from build123d import *

# Parameters (mm, degrees)
SKETCH1_W           = 102.2
SKETCH1_H           = 67.6
SKETCH1_R           = 1.6
BOSS_EXTRUDE1_DEPTH = 6
SKETCH2_W           = 138.2
SKETCH2_H           = 67.6
SKETCH2_R           = 2.5
BOSS_EXTRUDE2_DEPTH = 3.2
FILLET1_R           = 6
FILLET2_R           = 5
FILLET3_R           = 5


with BuildPart() as part:
    # Sketch1 → Boss-Extrude1 (new body)
    with BuildSketch(Plane.XY):
        with Locations((51.1, 33.8)):
            Rectangle(SKETCH1_W, SKETCH1_H)
        with BuildLine():
            Line((94.706674091, 2.5), (7.493325909, 2.5))
            ThreePointArc((7.493325909, 2.5), (7.045584412, 7.045584412), (2.5, 7.493325909))
            Line((2.5, 7.493325909), (2.5, 65.1))
            Line((2.5, 65.1), (99.7, 65.1))
            Line((99.7, 65.1), (99.7, 57.093325909))
            ThreePointArc((99.7, 57.093325909), (94.1, 54.1), (99.7, 51.106674091))
            Line((99.7, 51.106674091), (99.7, 7.493325909))
            ThreePointArc((99.7, 7.493325909), (95.154415588, 7.045584412), (94.706674091, 2.5))
        make_face(mode=Mode.SUBTRACT)
        with Locations((4.5, 4.5)):
            Circle(SKETCH1_R, mode=Mode.SUBTRACT)
        with Locations((97.7, 4.5)):
            Circle(SKETCH1_R, mode=Mode.SUBTRACT)
        with Locations((97.7, 54.1)):
            Circle(SKETCH1_R, mode=Mode.SUBTRACT)
    extrude(amount=BOSS_EXTRUDE1_DEPTH)

    # Sketch2 → Boss-Extrude2 (add)
    with BuildSketch(Plane(origin=(0, 0, 0), x_dir=(-1, 0, 0), z_dir=(0, 0, -1))):
        with Locations((-51.1, 33.8)):
            Rectangle(SKETCH2_W, SKETCH2_H)
        with Locations((-112.2, 59.6)):
            Circle(SKETCH2_R, mode=Mode.SUBTRACT)
        with Locations((-112.2, 8)):
            Circle(SKETCH2_R, mode=Mode.SUBTRACT)
        with Locations((10, 8)):
            Circle(SKETCH2_R, mode=Mode.SUBTRACT)
        with Locations((10, 59.6)):
            Circle(SKETCH2_R, mode=Mode.SUBTRACT)
    extrude(amount=BOSS_EXTRUDE2_DEPTH)

    # Fillet1
    fillet1_edges = [part.edges().sort_by_distance(p)[0] for p in [
        (120.2, 67.6, -1.6),
        (120.2, 0, -1.6),
        (-18, 0, -1.6),
        (-18, 67.6, -1.6),
    ]]
    fillet(fillet1_edges, radius=FILLET1_R)

    # Fillet2
    fillet2_edges = [part.edges().sort_by_distance(p)[0] for p in [
        (99.7, 51.106674091, 3),
        (99.7, 57.093325909, 3),
    ]]
    fillet(fillet2_edges, radius=FILLET2_R)

    # Fillet3
    fillet3_edges = [part.edges().sort_by_distance(p)[0] for p in [
        (7.493325909, 2.5, 3),
        (94.706674091, 2.5, 3),
        (99.7, 7.493325909, 3),
        (2.5, 7.493325909, 3),
    ]]
    fillet(fillet3_edges, radius=FILLET3_R)


solid = part.part
CAD build for the part. Positions are in the model's coordinates, mm. A direction names the side the tool comes from. Round coordinates to 2 decimals unless told otherwise and drop trailing zeros. Order: outer loops, then holes, each group sorted by start corner. A loop starts at its lowest first (then second) coordinate and runs counter-clockwise, first axis right, second up. Notation, with made-up numbers: M 55.5,34 L 96.5,34 A23 ccw 96.5,70 Z; hole C 31,-3 d11. An arc over 180 degrees is marked long. Use one line per item in the form item = value.
Q1. Saw through at A-A on x = -10. Give the cut face in (y, z).
Recorded:
outline = M 0,-3.2 L 5.5,-3.2 L 5.5,0 L 0,0 Z; M 10.5,-3.2 L 57.1,-3.2 L 57.1,0 L 10.5,0 Z; M 62.1,-3.2 L 67.6,-3.2 L 67.6,0 L 62.1,0 Z
Q2. Which spindle directions (+Z, -Z, +X, -X, +Y, -Y) get a long thin tool onto all of the face, cutting with end or side? Do faces 5 (the flat face through (111, 34, 0)), 6 (the cylindrical face through (3.4, 9.7, 3)), 7 (the flat face through (52, 0, 1)), 8 (the flat face through (-9, 34, 0)). Say none if no direction does.
Recorded:
face_5 = +Z, +X, +Y, -Y
face_6 = +Z
face_7 = +Z, -Z, +X, -X, -Y
face_8 = +Z, -X, +Y, -Y
Q3. Saw through at D-D on y = 59.6. Give the cut face in (x, z).
Recorded:
outline = M -18,-3.2 L -12.5,-3.2 L -12.5,0 L -18,0 Z; M -7.5,-3.2 L 109.7,-3.2 L 109.7,0 L 102.2,0 L 102.2,6 L 99,6 L 99,0 L 2.5,0 L 2.5,6 L 0,6 L 0,0 L -7.5,0 Z; M 114.7,-3.2 L 120.2,-3.2 L 120.2,0 L 114.7,0 Z
Q4. Flat gauge pins, fed straight in: P1, Ø3, axis at y = 34, z = 3.5, coming from the +X side; P2, Ø1, axis at x = 97.5, y = 53.5, coming from the +Z side; P3, Ø5, axis at y = 30, z = 3, coming from the -X side; P4, Ø3.5, axis at x = 97.7, y = 54.1, coming from the +Z side. Where does each tip first touch, or does it go through?
Recorded:
P1 = 102.2
P2 = 0
P3 = 0
P4 = 6
Q5. Saw through at B-B on z = 1.25. Give the cut face in (x, y).
Recorded:
outline = M 0,0 L 102.2,0 L 102.2,67.6 L 0,67.6 Z; hole M 2.5,12.56 A5 ccw 5.76,7.87 A3.6 cw 7.87,5.76 A5 ccw 12.56,2.5 L 89.64,2.5 A5 ccw 94.33,5.76 A3.6 cw 96.44,7.87 A5 ccw 99.7,12.56 L 99.7,46.04 A5 ccw 96.44,50.73 A3.6 cw 96.44,57.47 A5 ccw 99.7,62.16 L 99.7,65.1 L 2.5,65.1 Z; hole C 4.5,4.5 d3.2; hole C 97.7,4.5 d3.2; hole C 97.7,54.1 d3.2
Q6. Two-plate mould, pull along Y, no slides. Class faces 1 (the cylindrical face through (118.489, 65.796, -1.622)), 2 (the flat face through (120.2, 33, -2)), 3 (the flat face through (98, 5, 0)), 4 (the flat face through (50, 65.1, 3)): +Y half, -Y half, draft (parallel to the pull), parting line (faces both ways), or undercut.
Recorded:
face_1 = +Y half
face_2 = draft
face_3 = undercut
face_4 = undercut
Q7. Saw through at C-C on y = 26.5. Give the cut face in (x, z), then the cut area to 3 significant figures.
Recorded:
outline = M -18,-3.2 L 120.2,-3.2 L 120.2,0 L 102.2,0 L 102.2,6 L 99.7,6 L 99.7,0 L 2.5,0 L 2.5,6 L 0,6 L 0,0 L -18,0 Z
area = 472 mm^2
Q8. Probe L1, parallel to Y at x = -10, z = -1.25; L2, parallel to X at y = 16, z = 1.25; L3, parallel to Y at x = 54, z = 0.75. List the from-to ranges inside material, lowest first.
Recorded:
L1 = 0 to 5.5, 10.5 to 57.1, 62.1 to 67.6
L2 = 0 to 2.5, 99.7 to 102.2
L3 = 0 to 2.5, 65.1 to 67.6
